from build123d import *

# Parameters (mm, degrees)
CROQUIS1_R              = 1.25
SALIENTE_EXTRUIR2_DEPTH = 10
CROQUIS2_W              = 15
CROQUIS2_H              = 15
CROQUIS2_R              = 1.5
SALIENTE_EXTRUIR3_DEPTH = 4
CROQUIS3_R              = 2.85
CORTAR_EXTRUIR1_DEPTH   = 1.65
CORTAR_EXTRUIR2_REACH   = 173.683
CROQUIS4_W              = 4
CROQUIS4_H              = 10
CORTAR_EXTRUIR3_REACH   = 105.682
REDONDEO1_R             = 5
CORTAR_EXTRUIR5_DEPTH   = 5
CROQUIS8_W              = 52.105263158
CROQUIS8_H              = 60
CORTAR_EXTRUIR6_DEPTH   = 5
REDONDEO2_R             = 5


with BuildPart() as part:
    # Croquis1 → Saliente-Extruir2 (new body)
    with BuildSketch(Plane.XY):
        Polygon((-45, -90), (41, -90), (41, -75), (45, -75), (45, 75), (41, 75), (41, 90), (-45, 90), align=None)
        with Locations((-33.5, -83)):
            Circle(CROQUIS1_R, mode=Mode.SUBTRACT)
        with Locations((-33.5, -7)):
            Circle(CROQUIS1_R, mode=Mode.SUBTRACT)
        with Locations((32.5, -83)):
            Circle(CROQUIS1_R, mode=Mode.SUBTRACT)
        with Locations((32.5, -7)):
            Circle(CROQUIS1_R, mode=Mode.SUBTRACT)
        with Locations((-18, 3.533333333)):
            Circle(CROQUIS1_R, mode=Mode.SUBTRACT)
        with BuildLine():
            ThreePointArc((-14.3581, 61.783333333), (-13.3581, 62.783333333), (-12.3581, 61.783333333))
            Line((-12.3581, 61.783333333), (-12.3581, 3.283333333))
            ThreePointArc((-12.3581, 3.283333333), (-13.3581, 2.283333333), (-14.3581, 3.283333333))
            Line((-14.3581, 3.283333333), (-14.3581, 61.783333333))
        make_face(mode=Mode.SUBTRACT)
        with BuildLine():
            ThreePointArc((-9.9681, 61.783333333), (-8.9681, 62.783333333), (-7.9681, 61.783333333))
            Line((-7.9681, 61.783333333), (-7.9681, 3.283333333))
            ThreePointArc((-7.9681, 3.283333333), (-8.9681, 2.283333333), (-9.9681, 3.283333333))
            Line((-9.9681, 3.283333333), (-9.9681, 61.783333333))
        make_face(mode=Mode.SUBTRACT)
        with BuildLine():
            ThreePointArc((-5.5781, 61.783333333), (-4.5781, 62.783333333), (-3.5781, 61.783333333))
            Line((-3.5781, 61.783333333), (-3.5781, 3.283333333))
            ThreePointArc((-3.5781, 3.283333333), (-4.5781, 2.283333333), (-5.5781, 3.283333333))
            Line((-5.5781, 3.283333333), (-5.5781, 61.783333333))
        make_face(mode=Mode.SUBTRACT)
        with BuildLine():
            Line((-27.5, 81.033333333), (-27.5, 4))
            ThreePointArc((-27.5, 4), (-31.5, 0), (-35.5, 4))
            Line((-35.5, 4), (-35.5, 81.033333333))
            ThreePointArc((-35.5, 81.033333333), (-31.5, 85.033333333), (-27.5, 81.033333333))
        make_face(mode=Mode.SUBTRACT)
        with Locations((-18, 61.533333333)):
            Circle(CROQUIS1_R, mode=Mode.SUBTRACT)
        with BuildLine():
            ThreePointArc((-1.1881, 61.783333333), (-0.1881, 62.783333333), (0.8119, 61.783333333))
            Line((0.8119, 61.783333333), (0.8119, 3.283333333))
            ThreePointArc((0.8119, 3.283333333), (-0.1881, 2.283333333), (-1.1881, 3.283333333))
            Line((-1.1881, 3.283333333), (-1.1881, 61.783333333))
        make_face(mode=Mode.SUBTRACT)
        with BuildLine():
            ThreePointArc((3.2019, 61.783333333), (4.2019, 62.783333333), (5.2019, 61.783333333))
            Line((5.2019, 61.783333333), (5.2019, 3.283333333))
            ThreePointArc((5.2019, 3.283333333), (4.2019, 2.283333333), (3.2019, 3.283333333))
            Line((3.2019, 3.283333333), (3.2019, 61.783333333))
        make_face(mode=Mode.SUBTRACT)
        with BuildLine():
            ThreePointArc((7.5919, 61.783333333), (8.5919, 62.783333333), (9.5919, 61.783333333))
            Line((9.5919, 61.783333333), (9.5919, 3.283333333))
            ThreePointArc((9.5919, 3.283333333), (8.5919, 2.283333333), (7.5919, 3.283333333))
            Line((7.5919, 3.283333333), (7.5919, 61.783333333))
        make_face(mode=Mode.SUBTRACT)
        with BuildLine():
            ThreePointArc((11.9819, 61.783333333), (12.9819, 62.783333333), (13.9819, 61.783333333))
            Line((13.9819, 61.783333333), (13.9819, 3.283333333))
            ThreePointArc((13.9819, 3.283333333), (12.9819, 2.283333333), (11.9819, 3.283333333))
            Line((11.9819, 3.283333333), (11.9819, 61.783333333))
        make_face(mode=Mode.SUBTRACT)
        with Locations((31, 3.533333333)):
            Circle(CROQUIS1_R, mode=Mode.SUBTRACT)
        with BuildLine():
            Line((18.3719, 61.783333333), (18.3719, 3.283333333))
            ThreePointArc((18.3719, 3.283333333), (17.3719, 2.283333333), (16.3719, 3.283333333))
            Line((16.3719, 3.283333333), (16.3719, 61.783333333))
            ThreePointArc((16.3719, 61.783333333), (17.3719, 62.783333333), (18.3719, 61.783333333))
        make_face(mode=Mode.SUBTRACT)
        with BuildLine():
            Line((22.7619, 61.783333333), (22.7619, 3.283333333))
            ThreePointArc((22.7619, 3.283333333), (21.7619, 2.283333333), (20.7619, 3.283333333))
            Line((20.7619, 3.283333333), (20.7619, 61.783333333))
            ThreePointArc((20.7619, 61.783333333), (21.7619, 62.783333333), (22.7619, 61.783333333))
        make_face(mode=Mode.SUBTRACT)
        with BuildLine():
            Line((27.1519, 61.783333333), (27.1519, 3.283333333))
            ThreePointArc((27.1519, 3.283333333), (26.1519, 2.283333333), (25.1519, 3.283333333))
            Line((25.1519, 3.283333333), (25.1519, 61.783333333))
            ThreePointArc((25.1519, 61.783333333), (26.1519, 62.783333333), (27.1519, 61.783333333))
        make_face(mode=Mode.SUBTRACT)
        with BuildLine():
            ThreePointArc((-18.25, 64.808333333), (-19.25, 65.808333333), (-18.25, 66.808333333))
            Line((-18.25, 66.808333333), (31.25, 66.808333333))
            ThreePointArc((31.25, 66.808333333), (32.25, 65.808333333), (31.25, 64.808333333))
            Line((31.25, 64.808333333), (-18.25, 64.808333333))
        make_face(mode=Mode.SUBTRACT)
        with BuildLine():
            ThreePointArc((-18.25, 68.838333333), (-19.25, 69.838333333), (-18.25, 70.838333333))
            Line((-18.25, 70.838333333), (31.25, 70.838333333))
            ThreePointArc((31.25, 70.838333333), (32.25, 69.838333333), (31.25, 68.838333333))
            Line((31.25, 68.838333333), (-18.25, 68.838333333))
        make_face(mode=Mode.SUBTRACT)
        with BuildLine():
            ThreePointArc((-18.25, 72.868333333), (-19.25, 73.868333333), (-18.25, 74.868333333))
            Line((-18.25, 74.868333333), (31.25, 74.868333333))
            ThreePointArc((31.25, 74.868333333), (32.25, 73.868333333), (31.25, 72.868333333))
            Line((31.25, 72.868333333), (-18.25, 72.868333333))
        make_face(mode=Mode.SUBTRACT)
        with BuildLine():
            ThreePointArc((-18.25, 76.898333333), (-19.25, 77.898333333), (-18.25, 78.898333333))
            Line((-18.25, 78.898333333), (31.25, 78.898333333))
            ThreePointArc((31.25, 78.898333333), (32.25, 77.898333333), (31.25, 76.898333333))
            Line((31.25, 76.898333333), (-18.25, 76.898333333))
        make_face(mode=Mode.SUBTRACT)
        with BuildLine():
            Line((-18.25, 82.928333333), (31.25, 82.928333333))
            ThreePointArc((31.25, 82.928333333), (32.25, 81.928333333), (31.25, 80.928333333))
            Line((31.25, 80.928333333), (-18.25, 80.928333333))
            ThreePointArc((-18.25, 80.928333333), (-19.25, 81.928333333), (-18.25, 82.928333333))
        make_face(mode=Mode.SUBTRACT)
        with Locations((31, 61.533333333)):
            Circle(CROQUIS1_R, mode=Mode.SUBTRACT)
    extrude(amount=SALIENTE_EXTRUIR2_DEPTH)

    # Croquis2 → Saliente-Extruir3 (add)
    with BuildSketch(Plane.XZ.offset(90)):
        with Locations((33.5, -7.5)):
            Rectangle(CROQUIS2_W, CROQUIS2_H)
        with Locations((36.8, -10.8)):
            Circle(CROQUIS2_R, mode=Mode.SUBTRACT)
        with Locations((30.2, -4.2)):
            Circle(CROQUIS2_R, mode=Mode.SUBTRACT)
    saliente_extruir3 = extrude(amount=-SALIENTE_EXTRUIR3_DEPTH)

    # Croquis3 → Cortar-Extruir1 (cut)
    with BuildSketch(Plane.XZ.offset(90)):
        with Locations(Location((30.2, -4.2, 0), (0, 0, 270))):
            Circle(CROQUIS3_R)
        with Locations(Location((36.8, -10.8, 0), (0, 0, 270))):
            Circle(CROQUIS3_R)
    cortar_extruir1 = extrude(amount=-CORTAR_EXTRUIR1_DEPTH, mode=Mode.SUBTRACT)

    # Simetría2: Saliente-Extruir3, Cortar-Extruir1 across plane
    add(saliente_extruir3.mirror(Plane.ZX))
    add(cortar_extruir1.mirror(Plane.ZX), mode=Mode.SUBTRACT)

    # Croquis4 → Cortar-Extruir2 (cut, up to next)
    with BuildSketch(Plane(origin=(0, 75, 0), x_dir=(1, 0, 0), z_dir=(0, 1, 0)), mode=Mode.PRIVATE) as cortar_extruir2_sk1:
        with Locations((43, -5)):
            Rectangle(CROQUIS4_W, CROQUIS4_H)
    cortar_extruir2_tool1 = extrude(cortar_extruir2_sk1.sketch, amount=-CORTAR_EXTRUIR2_REACH, mode=Mode.PRIVATE) & part.part
    add(cortar_extruir2_tool1.solids().sort_by_distance((43, 75, 5))[0], mode=Mode.SUBTRACT)

    # Croquis5 → Cortar-Extruir3 (cut, up to next)
    with BuildSketch(Plane.XY.offset(10), mode=Mode.PRIVATE) as cortar_extruir3_sk1:
        Polygon((-45, 90), (-25, 90), (-25, 0), (-39, 0), (-39, -90), (-45, -90), (-45, 0), align=None)
    cortar_extruir3_tool1 = extrude(cortar_extruir3_sk1.sketch, amount=-CORTAR_EXTRUIR3_REACH, mode=Mode.PRIVATE) & part.part
    add(cortar_extruir3_tool1.solids().sort_by_distance((-36.615385, 24.230769, 10))[0], mode=Mode.SUBTRACT)

    # Redondeo1
    redondeo1_edges = [part.edges().sort_by_distance(p)[0] for p in [
        (-39, 0, 5),
    ]]
    fillet(redondeo1_edges, radius=REDONDEO1_R)

    # Croquis7 → Cortar-Extruir5 (cut)
    with BuildSketch(Plane(origin=(0, 0, 0), x_dir=(-1, 0, 0), z_dir=(0, 0, -1))):
        Polygon((39, -75), (39, -90), (-26, -90), (-26, -75), (-41, -75), (-41, 75), (-26, 75), (-26, 90), (39, 90), (39, 75), align=None)
    extrude(amount=-CORTAR_EXTRUIR5_DEPTH, mode=Mode.SUBTRACT)

    # Croquis8 → Cortar-Extruir6 (cut)
    with BuildSketch(Plane.XY.offset(10)):
        with Locations((-0.5, -45)):
            Rectangle(CROQUIS8_W, CROQUIS8_H)
    extrude(amount=-CORTAR_EXTRUIR6_DEPTH, mode=Mode.SUBTRACT)

    # Redondeo2
    redondeo2_edges = [part.edges().sort_by_distance(p)[0] for p in [
        (-26.552631579, -75, 7.5),
        (-26.552631579, -15, 7.5),
        (25.552631579, -15, 7.5),
        (25.552631579, -75, 7.5),
    ]]
    fillet(redondeo2_edges, radius=REDONDEO2_R)


solid = part.part
Model file for the job. Use its own axes, mm. A direction names the side the tool comes from. Round coordinates to 2 decimals unless told otherwise and drop trailing zeros. Order: outer loops, then holes, each group sorted by start corner. A loop starts at its lowest first (then second) coordinate and runs counter-clockwise, first axis right, second up. Notation, with made-up numbers: M 24.25,50 L 39.25,50 A23 ccw 39.25,64 Z; hole C 11,4 d8. An arc over 180 degrees is marked long. Write each question's results on one line, items separated by ' | '. Start each with the question number.
(1) Drop flat-ended pins along their axis: pin 1 (4 mm diameter, centred on y = 24, z = 8, fed in from -X); pin 2 (3 mm diameter, centred on x = 31, z = -4.5, fed in from -Y); pin 3 (3.5 mm diameter, centred on x = 30.2, z = -4.2, fed in from +Y). Give the stop position or say it passes through.
(2) Saw through at A-A, the plane y = -66. Give the cut face in (x, z), then the cut area to 3 significant figures.
(3) Saw through at C-C, the plane x = -30.5. Give the cut face in (y, z).
(4) Probe probe 1 along Y at (x, z) = (32.5, 7); probe 2 along Y at (x, z) = (-33.5, 6.7); probe 3 along Z at (x, y) = (36.8, 87.65). List the from-to ranges inside material, lowest first. Write a range as from..to.
(5) Saw through at B-B, the plane y = 18. State how many separate pieces and enclosed holes the cut face has, then the cut area to 3 significant figures.
(6) Two-plate mould, pull along Z, no slides. Class faces 1 (the face through (31.63, -87.19, -3.75)), 2 (the face through (7, 14, 5)), 3 (the face through (32.603, -89.187, -5.732)), 4 (the face through (33, -86, -7)): pulls with the +Z half, pulls with the -Z half, needs draft (parallel to the pull), parting line crosses it, or undercut.
(7) Which spindle directions (+Z, -Z, +X, -X, +Y, -Y) get a long thin tool onto all of the face, cutting with end or side? Do faces 5 (the face through (34, 75, 2)), 6 (the face through (41, 0, 7)), 7 (the face through (25.553, -45, 8)). Say none if no direction does.
Established:
1) pin 1: stops at x = -25 | pin 2: stops at y = -88.35 | pin 3: stops at y = 88.35
2) outline: M -39,5 L -26.55,5 L -26.55,10 L -39,10 Z; M 25.55,5 L 41,5 L 41,10 L 25.55,10 Z | area: 139 mm^2
3) outline: M -90,5 L 0,5 L 0,10 L -90,10 Z
4) probe 1: y = -90..-84.25, -81.75..-8.25, -5.75..90 | probe 2: y = -90..-84.25, -81.75..-8.25, -5.75..0 | probe 3: z = -15..-12.3, -9.3..10
5) separate pieces: 11 | enclosed holes: 0 | area: 230 mm^2
6) face 1: undercut | face 2: pulls with the -Z half | face 3: undercut | face 4: needs draft
7) face 5: -Z, +X, -X | face 6: +Z, -Z, +X, +Y, -Y | face 7: +Z, -Z
